Check sheet for the modelled part. Datum: model origin and axes. Units: mm. Face numbers are marked on the shaded views. Give positions to 0.01 mm unless a question says otherwise; leave off trailing zeros. Order: outer loops, then holes, each group sorted by start corner. A loop starts at its lowest first (then second) coordinate and runs counter-clockwise, first axis right, second up. Notation, with made-up numbers: (23.25, 59) -> (32.25, 59) arc R24 cw to (32.25, 93) -> close; hole circle Ø5 at (27.5, 55). An arc over 180 degrees is marked (long way). Answer in a Markdown table with one row per item. Add a question column.
(1) Cross-section at B-B (x = 138). Record the cut outline in (y, z).
(2) Cross-section at D-D (x = 83). Record the cut outline in (y, z).
(3) Thickness scan on L1, parallel to Y at x = 151, z = 12.75; L2, parallel to X at y = 5, z = 12; L3, parallel to Z at x = 107, y = 74.5. Record the ranges inside material, lowest first. Write a range as [from, to].
(4) Release check for a two-part mould opening along X. For the marked faces 1 and 2 record: released by +X, released by -X, zero draft, split by the parting line, or undercut.
(5) Cross-section at C-C (z = 11.25). State how many separate pieces and enclosed holes the cut face has, then the cut area to 3 significant figures.
(6) Go/stop test with a flat-tipped pin: pin 1 (11 mm diameter, centred on x = 78.5, y = 67, fed in from +Z). Record where the tip stops, or that it passes through.
(7) Cross-section at A-A (y = 52). Record the cut outline in (x, z).
```python
from build123d import *

# Parameters (mm, degrees)
F0_W     = 160
F0_H     = 100
F0_W_2   = 15
F0_H_2   = 80
F1_DEPTH = 5
F2_W     = 10
F2_H     = 10
F3_DEPTH = 10


with BuildPart() as f1:
    # F0 (on Top) → F1 (new body)
    with BuildSketch(Plane.XY):
        with Locations((80, 50)):
            Rectangle(F0_W, F0_H)
        with Locations((17.5, 50)):
            Rectangle(F0_W_2, F0_H_2, mode=Mode.SUBTRACT)
        with Locations((42.5, 50)):
            Rectangle(F0_W_2, F0_H_2, mode=Mode.SUBTRACT)
        with Locations((67.5, 50)):
            Rectangle(F0_W_2, F0_H_2, mode=Mode.SUBTRACT)
        with Locations((92.5, 50)):
            Rectangle(F0_W_2, F0_H_2, mode=Mode.SUBTRACT)
        with Locations((117.5, 50)):
            Rectangle(F0_W_2, F0_H_2, mode=Mode.SUBTRACT)
        with Locations((142.5, 50)):
            Rectangle(F0_W_2, F0_H_2, mode=Mode.SUBTRACT)
    extrude(amount=F1_DEPTH)

    # F2 (on face) → F3 (join)
    with BuildSketch(Plane.XY.offset(5)):
        with Locations((5, 95)):
            Rectangle(F2_W, F2_H)
        with Locations((80, 95)):
            Rectangle(F2_W, F2_H)
        with Locations((155, 95)):
            Rectangle(F2_W, F2_H)
        with Locations((155, 50)):
            Rectangle(F2_W, F2_H)
        with Locations((80, 50)):
            Rectangle(F2_W, F2_H)
        with Locations((5, 50)):
            Rectangle(F2_W, F2_H)
        with Locations((5, 5)):
            Rectangle(F2_W, F2_H)
        with Locations((155, 5)):
            Rectangle(F2_W, F2_H)
        with Locations((80, 5)):
            Rectangle(F2_W, F2_H)
    extrude(amount=F3_DEPTH)


solid = f1.part
```
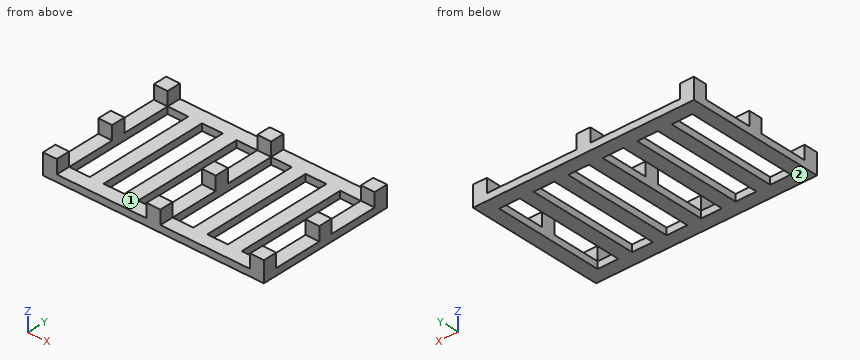
Answer below:
| question | item | result |
|---|---|---|
| 1 | outline | (0, 0) -> (10, 0) -> (10, 5) -> (0, 5) -> close; (90, 0) -> (100, 0) -> (100, 5) -> (90, 5) -> close |
| 2 | outline | (0, 0) -> (100, 0) -> (100, 15) -> (90, 15) -> (90, 5) -> (55, 5) -> (55, 15) -> (45, 15) -> (45, 5) -> (10, 5) -> (10, 15) -> (0, 15) -> close |
| 3 | L1 | y = [0, 10], [45, 55], [90, 100] |
| 3 | L2 | x = [0, 10], [75, 85], [150, 160] |
| 3 | L3 | z = [0, 5] |
| 4 | face 1 | undercut |
| 4 | face 2 | zero draft |
| 5 | separate pieces | 9 |
| 5 | enclosed holes | 0 |
| 5 | area | 900 mm² |
| 6 | pin 1 | stops at z = 5 |
| 7 | outline | (0, 0) -> (10, 0) -> (10, 15) -> (0, 15) -> close; (25, 0) -> (35, 0) -> (35, 5) -> (25, 5) -> close; (50, 0) -> (60, 0) -> (60, 5) -> (50, 5) -> close; (75, 0) -> (85, 0) -> (85, 15) -> (75, 15) -> close; (100, 0) -> (110, 0) -> (110, 5) -> (100, 5) -> close; (125, 0) -> (135, 0) -> (135, 5) -> (125, 5) -> close; (150, 0) -> (160, 0) -> (160, 15) -> (150, 15) -> close |
